Could you check a few things on this model? Use its own coordinates, in mm. A direction names the side the tool comes from. Coordinates: 2 decimals unless noted, no trailing zeros. Write each loop counter-clockwise with the first axis right and the second up, starting at its lowest first coordinate (ties: lowest second). Pieces come first, ordered by that corner, then holes.
Autodesk Inventor part; units mm, degrees
ref_plane "YZ Plane" through (0, 0, 0) normal (1, 0, 0) x (0, 1, 0)
ref_plane "XZ Plane" through (0, 0, 0) normal (0, 1, 0) x (-1, 0, 0)
ref_plane "XY Plane" through (0, 0, 0) normal (0, 0, 1) x (1, 0, 0)
sketch "スケッチ1" plane through (0, 0, 0) normal (0, 0, 1) x (1, 0, 0)
  line L0 (0, 0) -> (23.9, 0)
  line L1 (23.9, 0) -> (23.9, 8)
  line L2 (23.9, 8) -> (0, 8)
  line L3 (0, 8) -> (0, 0)
  line L4 (0, 0) -> (11, 0)
  line L5 (11, 0) -> (11, 3)
  line L6 (11, 3) -> (0, 3)
  line L7 (0, 3) -> (0, 0)
  line L8 (23.9, 0) -> (12.9, 0)
  line L9 (12.9, 0) -> (12.9, 3)
  line L10 (12.9, 3) -> (23.9, 3)
  line L11 (23.9, 3) -> (23.9, 0)
  line L12 (9, 8) -> (14.9, 8)
  line L13 (14.9, 8) -> (14.9, 0)
  line L14 (14.9, 0) -> (9, 0)
  line L15 (9, 0) -> (9, 8)
  line L16 (9, 8) -> (8, 8)
  line L17 (8, 8) -> (8, 4)
  line L18 (8, 4) -> (9, 4)
  line L19 (9, 4) -> (9, 8)
  line L20 (14.9, 8) -> (15.9, 8)
  line L21 (15.9, 8) -> (15.9, 4)
  line L22 (15.9, 4) -> (14.9, 4)
  line L23 (14.9, 4) -> (14.9, 8)
  dimension "d0" = 8
  dimension "d1" = 23.9
  dimension "d2" = 11
  dimension "d3" = 3
  dimension "d4" = 11
  dimension "d5" = 3
  dimension "d6" = 2
  dimension "d7" = 2
  dimension "d8" = 1
  dimension "d9" = 4
  dimension "d10" = 1
  dimension "d11" = 4
revolve "回転1" add sketch "スケッチ1" angle 360 about axis through (0, 0, 0) along (1, 0, 0) contours L3 L2 L17 L18 L15 L6 | L5 L6 L15 L2 L13 L10 L9 L0 | L13 L22 L21 L2 L1 L10
properties part number "Coupling_SOH_16C_6_6" material "アルミニウム 6061"
1. On a 3-axis mill with a long thin cutter (end or side, diameter ignored), from which of +Z, -Z, +X, -X, +Y, -Y can I reach the whole of each face in a straight line? I mean faces 4 (the face through (11, 0, 0)), 5 (the face through (15.9, -4, -2)), 6 (the face through (12.9, 0, 0)). Say none if no direction works.
Verdict:
face 4: -X
face 5: none
face 6: +X
2. For pin 1 (4 mm diameter, centred on x = 9.5, y = 3.5, fed in from +Z); pin 2 (1 mm diameter, centred on x = 2.5, z = 3.5, fed in from +Y); pin 3 (3.5 mm diameter, centred on y = 0, z = 0, fed in from -X), each with a flat end and sliding along its axis, tell me the tip position at first contact or that it passes through.
Verdict:
pin 1: stops at z = 7.86
pin 2: stops at y = 7.42
pin 3: stops at x = 11
3. Please list where these lines run through material, in increasing order: line 1 along X through (y, z) = (-4, 6); line 2 along Z through (x, y) = (8.5, 0); line 3 along Z through (x, y) = (20.75, 0).
Verdict:
line 1: x = 0 to 8, 9 to 14.9, 15.9 to 23.9
line 2: z = -4 to -3, 3 to 4
line 3: z = -8 to -3, 3 to 8
4. I want a section at C-C on x = 13.25. Please give me the cut outline in (y, z), plus the area to 3 significant figures.
Verdict:
outline: circle Ø16 at (0, 0); hole circle Ø6 at (0, 0)
area: 173 mm2
5. If we mould it in two halves opening along Y, with no side actions, what happens to faces 1 (the face through (8, -4, -2)), 2 (the face through (18, -3, 0)), 3 (the face through (15.393, -0.867, 3.905))? For each: pulls with the +Y half, pulls with the -Y half, needs draft (parallel to the pull), parting line crosses it, or undercut.
Verdict:
face 1: needs draft
face 2: undercut
face 3: parting line crosses it
6. I want a section at A-A on z = 0. Please give me the cut outline in (x, y).
Verdict:
outline: (0, -8) - (8, -8) - (8, -4) - (9, -4) - (9, -8) - (14.9, -8) - (14.9, -4) - (15.9, -4) - (15.9, -8) - (23.9, -8) - (23.9, -3) - (12.9, -3) - (12.9, 3) - (23.9, 3) - (23.9, 8) - (15.9, 8) - (15.9, 4) - (14.9, 4) - (14.9, 8) - (9, 8) - (9, 4) - (8, 4) - (8, 8) - (0, 8) - (0, 3) - (11, 3) - (11, -3) - (0, -3) - close
7. I want a section at D-D on z = -4.5. Please give me the cut outline in (x, y), plus the area to 3 significant figures.
Verdict:
outline: (0, -6.61) - (8, -6.61) - (8, 6.61) - (0, 6.61) - close; (9, -6.61) - (14.9, -6.61) - (14.9, 6.61) - (9, 6.61) - close; (15.9, -6.61) - (23.9, -6.61) - (23.9, 6.61) - (15.9, 6.61) - close
area: 290 mm2
